from build123d import *

# Parameters (mm, degrees)
F1_DEPTH = 50
F2_R     = 1.55
F3_DEPTH = 4


with BuildPart() as f1:
    # F0 (on Front) → F1 (new body)
    with BuildSketch(Plane.XZ):
        Polygon((60, 0), (0, 0), (0, -35), (4, -35), (4, -4), (60, -4), align=None)
    extrude(amount=F1_DEPTH)

    # F2 (on face) → F3 (cut, through all)
    with BuildSketch(Plane.XY):
        with Locations((40, -15)):
            Circle(F2_R)
        with Locations((20, -15)):
            Circle(F2_R)
        with Locations((20, -35)):
            Circle(F2_R)
        with Locations((40, -35)):
            Circle(F2_R)
        with Locations((13, -38)):
            Circle(F2_R)
        with Locations((13, -15)):
            Circle(F2_R)
        with Locations((53.38319, -9.517766)):
            Circle(F2_R)
    extrude(amount=-F3_DEPTH, mode=Mode.SUBTRACT)


solid = f1.part
Can you work these out from the model? Positions are in its coordinate system, mm. A direction names the side the tool comes from. Coordinates: 2 decimals unless noted, no trailing zeros. Loops run counter-clockwise (first coordinate to the right, second up) from the corner with the lowest first, then second, coordinate; pieces in that order, holes last. Notation, with made-up numbers: (64, 63.25) - (84, 63.25) arc R21 cw to (84, 85.25) - close; hole circle Ø5 at (-31, 88). An arc over 180 degrees is marked (long way). Put each result on its own line as item: value. Start each with the question number.
Item 1: Suppose I cut it at C-C (y = -15). Please give me the cut outline in (x, z).
Item 2: If I drill on line 1 along Y through (x, z) = (40, -1.95); line 2 along X through (y, z) = (-21, -25.5); line 3 along Z through (x, y) = (50, -29), over which ranges is the centre line in solid material (lowest first)?
Item 3: If we mould it in two halves opening along X, with no side actions, what happens to faces 3 (the face through (4, -25, -20)), 4 (the face through (2, -25, -35)), 5 (the face through (12.664, -39.513, -1.972)), 6 (the face through (0, -25, -17))? For each: +X half, -X half, draft (parallel to the pull), parting line (faces both ways), or undercut.
Item 4: Suppose I cut it at A-A (y = -35). Please give me the cut outline in (x, z), and give its area (3 significant figures).
Item 5: Suppose I cut it at B-B (x = 13). Please give me the cut outline in (y, z).
Item 6: For pin 1 (5 mm diameter, centred on x = 48, y = -37.5, fed in from -Z); pin 2 (12 mm diameter, centred on x = 38.5, y = -35, fed in from +Z); pin 3 (3 mm diameter, centred on y = -18, z = -8, fed in from +X), each with a flat end and sliding along its axis, tell me the tip position at first contact or that it passes through.
Item 7: Suppose I cut it at D-D (y = -23). Please give me the cut outline in (x, z).
Item 8: Which directions (+Z, -Z, +X, -X, +Y, -Y) give clear straight access to the entire face, cutting with the end or side of a thin tool? Please do faces 1 (the face through (32, -25, -4)), 2 (the face through (17, -50, -3)).
Here are the results:
1. outline: (0, -35) - (4, -35) - (4, -4) - (11.45, -4) - (11.45, 0) - (0, 0) - close; (14.55, -4) - (18.45, -4) - (18.45, 0) - (14.55, 0) - close; (21.55, -4) - (38.45, -4) - (38.45, 0) - (21.55, 0) - close; (41.55, -4) - (60, -4) - (60, 0) - (41.55, 0) - close
2. line 1: -50 to -36.55, -33.45 to -16.55, -13.45 to 0
2. line 2: 0 to 4
2. line 3: -4 to 0
3. face 3: +X half
3. face 4: draft
3. face 5: undercut
3. face 6: -X half
4. outline: (0, -35) - (4, -35) - (4, -4) - (18.45, -4) - (18.45, 0) - (0, 0) - close; (21.55, -4) - (38.45, -4) - (38.45, 0) - (21.55, 0) - close; (41.55, -4) - (60, -4) - (60, 0) - (41.55, 0) - close
4. area: 339 mm²
5. outline: (-50, -4) - (-39.55, -4) - (-39.55, 0) - (-50, 0) - close; (-36.45, -4) - (-16.55, -4) - (-16.55, 0) - (-36.45, 0) - close; (-13.45, -4) - (0, -4) - (0, 0) - (-13.45, 0) - close
6. pin 1: z = -4
6. pin 2: z = 0
6. pin 3: x = 4
7. outline: (0, -35) - (4, -35) - (4, -4) - (60, -4) - (60, 0) - (0, 0) - close
8. face 1: -Z, +X, +Y, -Y
8. face 2: +Z, -Z, +X, -X, -Y
